Build history of the part. All positions in model axes, mm. A direction names the side the tool comes from. Round coordinates to 2 decimals unless told otherwise and drop trailing zeros. Use CSV: the item, a comma, the result in double quotes.
from build123d import *

# Parameters (mm, degrees)
F_1_FR_W        = 162.591921451
F_1_FR_H        = 106.952100423
F_1_FR_R        = 3.052899236
EXTRUDE_1_DEPTH = 10


with BuildPart() as part:
    # Эскиз1_fr → Бобышка-Вытянуть1 (new body)
    with BuildSketch(Plane.XY):
        with Locations((41.575310714, -4.636651753)):
            Rectangle(F_1_FR_W, F_1_FR_H)
        with Locations((-22.101373353, 28.438130748)):
            Circle(F_1_FR_R, mode=Mode.SUBTRACT)
        with BuildLine():
            ThreePointArc((-26.934111294, 37.298150306), (-31.783615034, 31.28584889), (-30.961392911, 23.605392807))
            ThreePointArc((-30.961392911, 23.605392807), (-27.778379385, 22.669212359), (-26.842198936, 25.852225885))
            ThreePointArc((-26.842198936, 25.852225885), (-27.282154135, 29.961889802), (-24.687278216, 33.178956331))
            ThreePointArc((-24.687278216, 33.178956331), (-23.751097767, 36.361969857), (-26.934111294, 37.298150306))
        make_face(mode=Mode.SUBTRACT)
    extrude(amount=EXTRUDE_1_DEPTH)


solid = part.part
(1) Wall check: line 1 (X direction, y = 28, z = 6.25); line 2 (X direction, y = 31, z = 3.75); line 3 (Y direction, x = -28, z = 6.75). Give the ranges that are in metal, low to high. Write a range as from..to.
Answer block:
line 1,"x = -39.72..-32.18, -27.48..-25.12, -19.08..122.87"
line 2,"x = -39.72..-31.86, -26.86..-23.76, -20.44..122.87"
line 3,"y = -58.11..22.56, 36.63..48.84"
(2) Two-plate mould, pull along Y, no slides. Class faces 1 (the face through (40, 48.839, 5)), 2 (the face through (40, -4, 0)), 3 (the face through (-31.752, 31.392, 4.93)): released by +Y, released by -Y, zero draft, split by the parting line, or undercut.
Answer block:
face 1,"released by +Y"
face 2,"zero draft"
face 3,"undercut"
(3) Drop a flat-ended pin along its axis: pin 1 (2 mm diameter, centred on x = 30.5, y = -8, fed in from -Z). Give the stop position or say it passes through.
Answer block:
pin 1,"stops at z = 0"
(4) Tool access for faces 4 (the face through (122.871, -5, 5)), 5 (the face through (-27.3, 29.9, 4.9)): list every direction of +Z, -Z, +X, -X, +Y, -Y with a clear straight run to the whole face (end or side of a thin tool).
Answer block:
face 4,"+Z, -Z, +X, +Y, -Y"
face 5,"+Z, -Z"
